For this review, take the finished solid that the model builds, in its own axes (mm). A direction names the side the tool comes from. Give positions to 0.01 mm unless a question says otherwise; leave off trailing zeros. Write each loop counter-clockwise with the first axis right and the second up, starting at its lowest first coordinate (ties: lowest second). Pieces come first, ordered by that corner, then holes.
1) We need section A-A on z = -38. Give the boundary of the cut face in (x, y).
2) We need section B-B on y = 0.6. Give the boundary of the cut face in (x, z).
3) Draft analysis for pull direction Z (two halves, no side actions). For faces 4 (the face through (-10, 0, -30)), 5 (the face through (-8.95, 1.77, -12.54)), 6 (the face through (-14, 1, 0)), state which applies: pulls with the +Z half, pulls with the -Z half, needs draft (parallel to the pull), parting line crosses it, or undercut.
4) We need section C-C on x = -17. Give the boundary of the cut face in (y, z), and give its area (3 significant figures).
5) Wall thickness on line 1 along Z through (x, y) = (-10, 2.3); line 2 along X through (y, z) = (0.8, -10); line 3 along Z through (x, y) = (-8.75, 3.4): over which ranges is each line inside the solid? List them lowest first.
6) We need section D-D on z = -55.5. Give the boundary of the cut face in (x, y), and give its area (3 significant figures).
7) Machinability: for faces 1 (the face through (-10, 3.5, -57)), 2 (the face through (-7.5, 3, -55)), 3 (the face through (-12.5, 3, -4)), which of the approach directions +Z, -Z, +X, -X, +Y, -Y give a long, thin tool a straight path to every point of the face, cutting with its end or side? Answer none if there is none.
8) For P1, Ø1, axis at x = -4, z = -37.5, coming from the +Y side; P2, Ø0.8, axis at y = 3, z = -5, coming from the +X side; P3, Ø0.8, axis at y = 3, z = -30, coming from the -X side, all flat-tipped, find the tip position at first contact; note any pin that passes through.
Autodesk Inventor part; units mm, degrees
ref_plane "YZ Plane" through (0, 0, 0) normal (1, 0, 0) x (0, 1, 0)
ref_plane "XZ Plane" through (0, 0, 0) normal (0, 1, 0) x (-1, 0, 0)
ref_plane "XY Plane" through (0, 0, 0) normal (0, 0, 1) x (1, 0, 0)
sketch "Sketch1" plane through (0, 0, 0) normal (0, 1, 0) x (-1, 0, 0)
  line L0 (0, 0) -> (20, 0)
  line L1 (20, 0) -> (20, -60)
  line L2 (20, -60) -> (0, -60)
  line L3 (0, -60) -> (0, 0)
  dimension "d0" = 20
  dimension "d1" = 60
extrude "Extrusion1" add sketch "Sketch1" along normal blind 2
sketch "Sketch2" plane through (0, 2, 0) normal (0, 1, 0) x (1, 0, 0)
  line L0 (0, 60) -> (-20, 60)
  line L1 (-7.5, 0) -> (-12.5, 0)
  line L2 (-12.5, 0) -> (-12.5, 60)
  line L3 (-12.5, 60) -> (-7.5, 60)
  line L4 (-7.5, 60) -> (-7.5, 0)
  line L5 (-7.5, 0) -> (-12.5, 60) construction
  line L6 (-12.5, 0) -> (-7.5, 60) construction
  point P0 (0, 0)
  point P1 (-10, 30)
  dimension "d4" = 5
extrude "Extrusion2" add sketch "Sketch2" along normal blind 1.5
fillet "Fillet1" radius 10 2 edges at (0, 1, 0) (0, 1, -60)
sketch "Sketch3" plane through (0, 0, 0) normal (0, -1, 0) x (1, 0, 0)
  point P0 (0, 0)
  point P1 (-10, -50)
  point P2 (-10, -10)
hole "Hole1" at (-10, 0, -50) at (-10, 0, -10) direction (0, 1, 0) diameter 5.5 end through all
properties part number "gap filler y axis"
Results list:
1. outline: (-20, 0) - (0, 0) - (0, 2) - (-7.5, 2) - (-7.5, 3.5) - (-12.5, 3.5) - (-12.5, 2) - (-20, 2) - close
2. outline: (-20, -60) - (-10, -60) arc R10 ccw to (0, -50) - (0, -10) arc R10 ccw to (-10, 0) - (-20, 0) - close; hole circle Ø5.5 at (-10, -50); hole circle Ø5.5 at (-10, -10)
3. face 4: needs draft
3. face 5: undercut
3. face 6: pulls with the +Z half
4. outline: (0, -60) - (2, -60) - (2, 0) - (0, 0) - close
4. area: 120 mm2
5. line 1: z = -60 to -52.75, -47.25 to -12.75, -7.25 to 0
5. line 2: x = -20 to -12.75, -7.25 to 0
5. line 3: z = -59.92 to -52.45, -47.55 to -12.45, -7.55 to -0.08
6. outline: (-20, 0) - (-1.65, 0) - (-1.65, 2) - (-7.5, 2) - (-7.5, 3.5) - (-12.5, 3.5) - (-12.5, 2) - (-20, 2) - close
6. area: 44.2 mm2
7. face 1: +Z, -Z, +X, -X, +Y
7. face 2: +Z, -Z, +X, +Y
7. face 3: +Z, -Z, -X, +Y
8. P1: stops at y = 2
8. P2: stops at x = -7.5
8. P3: stops at x = -12.5
